Geometry: final body of the model. Coordinates: model frame, mm. A direction names the side the tool comes from. Round coordinates to 2 decimals unless told otherwise and drop trailing zeros. Loops run counter-clockwise (first coordinate to the right, second up) from the corner with the lowest first, then second, coordinate; pieces in that order, holes last. Notation, with made-up numbers: (16, 51.5) - (40, 51.5) arc R24 cw to (40, 76.5) - close; hole circle Ø11 at (9.5, 89.25). An arc over 180 degrees is marked (long way). Answer as a JSON object with one key per item and string values. Group by question number.
Item 1: Section B-B (y = -18). Return the cut outline in (x, z), plus the area to 3 significant figures.
Item 2: Section C-C (x = 21). Return the cut outline in (y, z).
Item 3: First-contact query: pin 1 (6 mm diameter, centred on x = 26.5, y = -27.5, fed in from +Z); pin 2 (14.5 mm diameter, centred on x = 16.5, y = -11, fed in from -Z). Flat tips, straight axial feed; report the tip coordinate or a pass-through.
Item 4: Section A-A (y = -28.5). Return the cut outline in (x, z).
Item 5: Reachability of faces 3 (the face through (30.8, -16, 18)), 4 (the face through (0.76, -4.199, 42.715)), 5 (the face through (16, -16, 28)) from +Z, -Z, +X, -X, +Y, -Y: full face, straight path, thin tool, end or side. Return the list, or none.
Item 6: Line query: line 1 (Z direction, x = 0.35, y = -28.5); line 2 (Z direction, x = 31.15, y = -8.5); line 3 (Y direction, x = 31, z = 41). Output: solid intervals per line, ascending.
Item 7: Draft query along X for faces 1 (the face through (31.56, -0.285, 10.301)), 2 (the face through (30.8, -16, 35)). Return one class per face: released by +X, released by -X, zero draft, split by the parting line, or undercut.
```python
from build123d import *

# Parameters (mm, degrees)
F1_DEPTH = 33
F2_R     = 1.1
F2_R_2   = 2
F3_DEPTH = 32.301
F4_R     = 1


with BuildPart() as f1:
    # F0 (on Front) → F1 (new body)
    with BuildSketch(Plane.XZ):
        Polygon((0, 26.5), (0, 0), (1.5, 0), (1.5, 25), (30.8, 25), (30.8, 0), (32.3, 0), (32.3, 26.5), align=None)
    extrude(amount=F1_DEPTH)

    # F2 (on face) → F3 (cut, through all)
    with BuildSketch(Plane(origin=(0, 0, 0), x_dir=(0, -1, 0), z_dir=(-1, 0, 0))):
        with BuildLine():
            Line((0, 10), (0, 0))
            Line((0, 0), (33, 0))
            Line((33, 0), (33, 10))
            Line((33, 10), (12.5, 10))
            Line((12.5, 10), (12.5, 12))
            ThreePointArc((12.5, 12), (8.5, 16), (4.5, 12))
            Line((4.5, 12), (4.5, 10))
            Line((4.5, 10), (0, 10))
        make_face()
        with Locations((14.7225396744, 12)):
            Circle(F2_R)
        with Locations((12.9, 16.4)):
            Circle(F2_R)
        with Locations((8.5, 18.2225396744)):
            Circle(F2_R)
        with Locations((4.1, 16.4)):
            Circle(F2_R)
        with Locations((2.2774603256, 12)):
            Circle(F2_R)
        with Locations((28.5, 19)):
            Circle(F2_R_2)
    extrude(amount=-F3_DEPTH, mode=Mode.SUBTRACT)

    # F4
    f4_edges = [f1.edges().sort_by_distance(p)[0] for p in [
        (31.55, 0, 10),
        (0.75, 0, 10),
        (0.75, -12.5, 10),
        (31.55, -12.5, 10),
        (0.75, -4.5, 10),
        (31.55, -4.5, 10),
        (0.75, -33, 10),
        (31.55, -33, 10),
    ]]
    fillet(f4_edges, radius=F4_R)

    # F6: F1 across plane


with BuildPart() as f1_1:
    add(f1.part)
    add(f1.part.mirror(Plane.XY.offset(26.5)))


solid = f1_1.part
```
Values:
{
 "1": {"outline": "(0, 10) - (1.5, 10) - (1.5, 25) - (30.8, 25) - (30.8, 10) - (32.3, 10) - (32.3, 43) - (30.8, 43) - (30.8, 28) - (1.5, 28) - (1.5, 43) - (0, 43) - close", "area": "187 mm^2"},
 "2": {"outline": "(-33, 25) - (0, 25) - (0, 28) - (-33, 28) - close"},
 "3": {"pin 1": "stops at z = 28", "pin 2": "stops at z = 25"},
 "4": {"outline": "(0, 10) - (1.5, 10) - (1.5, 17) - (0, 17) - close; (0, 21) - (1.5, 21) - (1.5, 25) - (30.8, 25) - (30.8, 21) - (32.3, 21) - (32.3, 32) - (30.8, 32) - (30.8, 28) - (1.5, 28) - (1.5, 32) - (0, 32) - close; (0, 36) - (1.5, 36) - (1.5, 43) - (0, 43) - close; (30.8, 10) - (32.3, 10) - (32.3, 17) - (30.8, 17) - close; (30.8, 36) - (32.3, 36) - (32.3, 43) - (30.8, 43) - close"},
 "5": {"face 3": "-Z, +Y, -Y", "face 4": "+Z, +X, -X", "face 5": "+Z, +Y, -Y"},
 "6": {"line 1": "z = 10 to 17, 21 to 32, 36 to 43", "line 2": "z = 16 to 17.12, 19.32 to 33.68, 35.88 to 37", "line 3": "y = -33 to -15.82, -13.62 to -12.5, -4.5 to -3.38, -1.18 to 0"},
 "7": {"face 1": "zero draft", "face 2": "undercut"}
}
